```python
from build123d import *

# Parameters (mm, degrees)
F3_D     = 4.5
F3_DEPTH = 7
F3_TIP   = 1.3519363928


with BuildPart() as f1:
    # F0 (on Front) → F1 (revolve)
    with BuildSketch(Plane.XZ):
        Polygon((-12.7, 0), (-3, 0), (-3, 9.2), (-6, 9.2), (-6, 5), (-12.7, 5), align=None)
    revolve(axis=Axis((0, 0, 4.6), (0, 0, -1)))

    # F3
    with Locations(Plane.XY.offset(5)):
        with Locations((-4.75, 8.227241336), (-9.5, 0), (-4.75, -8.227241336), (4.75, -8.227241336), (9.5, 0), (4.75, 8.227241336)):
            Hole(F3_D / 2, depth=F3_DEPTH)
            with Locations((0, 0, -(F3_DEPTH + F3_TIP / 2))):  # 118° drill point
                Cone(0, F3_D / 2, F3_TIP, mode=Mode.SUBTRACT)


solid = f1.part
```
Build history of the part. All positions in model axes, mm. A direction names the side the tool comes from. Round coordinates to 2 decimals unless told otherwise and drop trailing zeros. Loops run counter-clockwise (first coordinate to the right, second up) from the corner with the lowest first, then second, coordinate; pieces in that order, holes last.
Item 1: Drill centre lines: line 1 along X through (y, z) = (-0.25, 4.75); line 2 along X through (y, z) = (-0.75, 0.5); line 3 along Y through (x, z) = (4.75, 1.05). Where is each one in solid material? Low to high.
Item 2: Saw through at C-C (z = 6.5). List the corners of the cut face in (x, y).
Item 3: Saw through at D-D (x = -4.75). List the corners of the cut face in (y, z).
Item 4: Saw through at A-A (x = 0). List the corners of the cut face in (y, z).
Item 5: Two-plate mould, pull along Y, no slides. Class faces 3 (the face through (-5.79, 6.23, 2.46)), 4 (the face through (2.75, -12.4, 2.46)), 5 (the face through (-3, -5.5, 5)): released by +Y, released by -Y, zero draft, split by the parting line, or undercut.
Item 6: Pin check, flat tips, straight feed: P1, Ø5, axis at x = -4.75, y = 8.23, coming from the +Z side; P2, Ø1.5, axis at x = 8, z = 1.5, coming from the -Y side; P3, Ø1.5, axis at y = -4.5, z = 6, coming from the -X side. Stop position of each tip, or through.
Item 7: Saw through at B-B (y = 0). List the corners of the cut face in (x, z), then the cut area to 3 significant figures.
Item 8: Which spindle directions (+Z, -Z, +X, -X, +Y, -Y) get a long thin tool onto all of the face, cutting with end or side? Do faces 1 (the face through (-7.252, 0.099, 2.465)), 2 (the face through (6, 0, 7)). Say none if no direction does.
Worked answers:
1. line 1: x = -12.7 to -11.74, -7.26 to -2.99, 2.99 to 7.26, 11.74 to 12.7
1. line 2: x = -12.68 to -11.62, -7.38 to -2.9, 2.9 to 7.38, 11.62 to 12.68
1. line 3: y = -11.78 to -10.48, -5.98 to 5.98, 10.48 to 11.78
2. outline: circle Ø12 at (0, 0); hole circle Ø6 at (0, 0)
3. outline: (-11.78, 0) - (-10.48, 0) - (-10.48, 5) - (-11.78, 5) - close; (-5.98, 0) - (5.98, 0) - (5.98, 5) - (3.67, 5) - (3.67, 9.2) - (-3.67, 9.2) - (-3.67, 5) - (-5.98, 5) - close; (10.48, 0) - (11.78, 0) - (11.78, 5) - (10.48, 5) - close
4. outline: (-12.7, 0) - (-3, 0) - (-3, 9.2) - (-6, 9.2) - (-6, 5) - (-12.7, 5) - close; (3, 0) - (12.7, 0) - (12.7, 5) - (6, 5) - (6, 9.2) - (3, 9.2) - close
5. face 3: undercut
5. face 4: split by the parting line
5. face 5: zero draft
6. P1: stops at z = 5
6. P2: stops at y = -10.43
6. P3: stops at x = -4.68
7. outline: (-12.7, 0) - (-11.75, 0) - (-11.75, 5) - (-12.7, 5) - close; (-7.25, 0) - (-3, 0) - (-3, 9.2) - (-6, 9.2) - (-6, 5) - (-7.25, 5) - close; (3, 0) - (7.25, 0) - (7.25, 5) - (6, 5) - (6, 9.2) - (3, 9.2) - close; (11.75, 0) - (12.7, 0) - (12.7, 5) - (11.75, 5) - close
7. area: 77.2 mm2
8. face 1: +Z, -Z
8. face 2: +Z
